from build123d import *

# Parameters (mm, degrees)
SKETCH2_R           = 6.35
SKETCH2_W           = 80.2259
SKETCH2_H           = 23.8252
SKETCH2_W_2         = 77.0509
SKETCH2_H_2         = 20.6502
BOSS_EXTRUDE1_DEPTH = 2
SKETCH5_R           = 1.5875
CUT_EXTRUDE1_DEPTH  = 2.54


with BuildPart() as part:
    # Sketch2 → Boss-Extrude1 (new body)
    # profile 1 of 7: a face of its own
    with BuildSketch(Plane.XY):
        with BuildLine():
            Line((-40.11295, -6.148361062), (-40.11295, 6.148361062))
            ThreePointArc((-40.11295, 6.148361062), (-44.87545, 0), (-40.11295, -6.148361062))
        make_face()
    # profile 2 of 7: a face of its own
    with BuildSketch(Plane.XY):
        with BuildLine():
            Line((-38.52545, -6.35), (-38.52545, 6.35))
            ThreePointArc((-38.52545, 6.35), (-39.325577257, 6.299388571), (-40.11295, 6.148361062))
            Line((-40.11295, 6.148361062), (-40.11295, -6.148361062))
            ThreePointArc((-40.11295, -6.148361062), (-39.325577257, -6.299388571), (-38.52545, -6.35))
        make_face()
    # profile 3 of 7: a face of its own
    with BuildSketch(Plane.XY):
        with Locations((-38.52545, 0)):
            Circle(SKETCH2_R)
    # profile 4 of 7: a face of its own
    with BuildSketch(Plane.XY):
        with Locations((-38.52545, 0)):
            Circle(SKETCH2_R)
    # profile 5 of 7: a face of its own
    with BuildSketch(Plane.XY):
        Rectangle(SKETCH2_W, SKETCH2_H)
        Rectangle(SKETCH2_W_2, SKETCH2_H_2, mode=Mode.SUBTRACT)
    # profile 6 of 7: a face of its own
    with BuildSketch(Plane.XY):
        Rectangle(SKETCH2_W_2, SKETCH2_H_2)
    # profile 7 of 7: a face of its own
    with BuildSketch(Plane.XY):
        with BuildLine():
            ThreePointArc((-32.17545, 0), (-34.035321939, 4.490128061), (-38.52545, 6.35))
            Line((-38.52545, 6.35), (-38.52545, -6.35))
            ThreePointArc((-38.52545, -6.35), (-34.035321939, -4.490128061), (-32.17545, 0))
        make_face()
    extrude(amount=BOSS_EXTRUDE1_DEPTH)

    # Sketch5 → Cut-Extrude1 (cut)
    with BuildSketch(Plane(origin=(0, 0, 0), x_dir=(-1, 0, 0), z_dir=(0, 0, -1))):
        with Locations((41.70045, 0)):
            Circle(SKETCH5_R)
    extrude(amount=-CUT_EXTRUDE1_DEPTH, mode=Mode.SUBTRACT)


solid = part.part
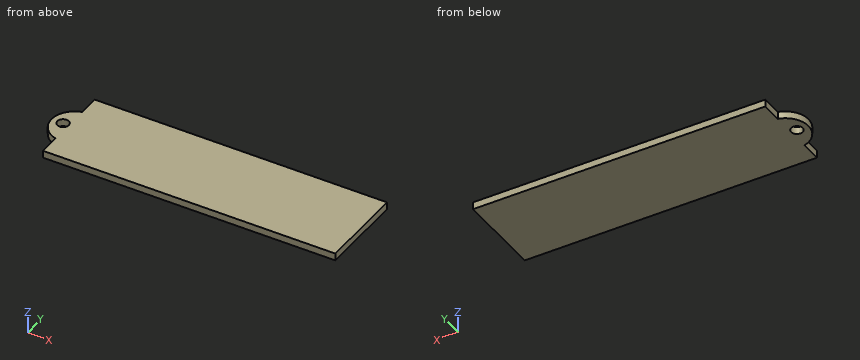
The model under review builds one solid part; all positions refer to its coordinate system, in mm. Give positions to 0.01 mm unless a question says otherwise; leave off trailing zeros. Order: outer loops, then holes, each group sorted by start corner. A loop starts at its lowest first (then second) coordinate and runs counter-clockwise, first axis right, second up. Notation, with made-up numbers: M 50.25,-23.75 L 83.25,-23.75 A22 cw 83.25,12.25 Z; hole C -31.75,-10 d11. An arc over 180 degrees is marked long. Answer in a Markdown table with one row per item. Add a question column.
1. Add section D-D on y = 5. State the section outline as (x, z) points, plus the area to 3 significant figures.
2. For pin 1 Ø1.9 at (x, y) = (-41.7, 0) entering from +Z; pin 2 Ø5 at (x, y) = (-36, -5) entering from -Z; pin 3 Ø0.6 at (y, z) = (10, 0.5) entering from -X, all flat-tipped, find the tip position at first contact; note any pin that passes through.
3. Add section C-C on y = 9.25. State the section outline as (x, z) points, plus the area to 3 significant figures.
4. Add section B-B on y = 0. State the section outline as (x, z) points.
5. To check wall thickness, follow line 1 along X through (y, z) = (9.5, 1.4); line 2 along Y through (x, z) = (-41, 0.9); line 3 along X through (y, z) = (-4.25, 1.55). State the ranges of each line that lie inside material, in increasing order.
The answers:
| question | item | result |
|---|---|---|
| 1 | outline | M -42.44,0 L 40.11,0 L 40.11,2 L -42.44,2 Z |
| 1 | area | 165 mm2 |
| 2 | pin 1 | through |
| 2 | pin 2 | z = 0 |
| 2 | pin 3 | x = -40.11 |
| 3 | outline | M -40.11,0 L 40.11,0 L 40.11,2 L -40.11,2 Z |
| 3 | area | 160 mm2 |
| 4 | outline | M -44.88,0 L -43.29,0 L -43.29,2 L -44.88,2 Z; M -40.11,0 L 40.11,0 L 40.11,2 L -40.11,2 Z |
| 5 | line 1 | -40.11 to 40.11 |
| 5 | line 2 | -5.85 to -1.42, 1.42 to 5.85 |
| 5 | line 3 | -43.24 to 40.11 |
